Could you check a few things on this model? Use its own coordinates, in mm. A direction names the side the tool comes from. Round coordinates to 2 decimals unless told otherwise and drop trailing zeros. Write each loop counter-clockwise with the first axis right and the second up, starting at its lowest first coordinate (ties: lowest second). Pieces come first, ordered by that corner, then holes. Notation, with made-up numbers: M 6,18 L 47,18 A9 cw 47,26 Z; hole C 11,45.5 d5. An arc over 180 degrees is marked long. One line per item, written item: value. Start each with the question number.
(1) I want a section at B-B on y = 18. Please give me the cut outline in (x, z), and give its area (3 significant figures).
(2) If I drill on L1, parallel to Y at x = 4, z = 4.5; L2, parallel to Y at x = 10.5, z = 1.75, over which ranges is the centre line in solid material (lowest first)?
(3) I want a section at A-A on z = 5.25. Count the separate pieces of the cut face and the enclosed holes in it, and give its area (3 significant figures).
(4) I'm going to push a flat-ended pin straight in: pin 1 Ø1 at (x, y) = (-10, -40) entering from -Z. Where does the tip first touch, or does it pass through?
(5) Thinking about a two-plate mould opening in X: for faces 4 (the face through (-69.947, -1, 5)), 5 (the face through (-6, -74, 0)), 6 (the face through (72.986, -73.297, 6.19)), which applies, released by +X, released by -X, zero draft, split by the parting line, or undercut?
(6) Which directions (+Z, -Z, +X, -X, +Y, -Y) give clear straight access to the entire face, cutting with the end or side of a thin tool? Please do faces 1 (the face through (-78, -77, 6)), 2 (the face through (1, -69.947, 5)), 3 (the face through (77.552, -1, 6)).
```python
from build123d import *

# Parameters (mm, degrees)
F1_DEPTH = 10.5
F3_DEPTH = 10
F5_DEPTH = 9
F6_R     = 2


with BuildPart() as f1:
    # F0 (on Top) → F1 (new body)
    with BuildSketch(Plane.XY):
        with BuildLine():
            Line((-74, -79), (59, -79))
            ThreePointArc((59, -79), (73.1421356237, -73.1421356237), (79, -59))
            Line((79, -59), (79, 59))
            ThreePointArc((79, 59), (73.1421356237, 73.1421356237), (59, 79))
            Line((59, 79), (-59, 79))
            ThreePointArc((-59, 79), (-73.1421356237, 73.1421356237), (-79, 59))
            Line((-79, 59), (-79, -74))
            ThreePointArc((-79, -74), (-77.5355339059, -77.5355339059), (-74, -79))
        make_face()
    extrude(amount=F1_DEPTH)

    # F2 (on face) → F3 (cut)
    with BuildSketch(Plane.XY.offset(10.5)):
        with BuildLine():
            Line((77.5522068143, -59), (77.5522068143, 59))
            ThreePointArc((77.5522068143, 59), (72.1183912444, 72.1183912444), (59, 77.5522068143))
            Line((59, 77.5522068143), (-59, 77.5522068143))
            ThreePointArc((-59, 77.5522068143), (-72.1183912444, 72.1183912444), (-77.5522068143, 59))
            Line((-77.5522068143, 59), (-77.5522068143, -59.0002068143))
            ThreePointArc((-77.5522068143, -59.0002068143), (-72.1184518189, -72.1184518189), (-59.0002068143, -77.5522068143))
            Line((-59.0002068143, -77.5522068143), (59, -77.5522068143))
            ThreePointArc((59, -77.5522068143), (72.1183912444, -72.1183912444), (77.5522068143, -59))
        make_face()
        with BuildLine():
            ThreePointArc((59, 70.9469467402), (67.4477670544, 67.4477670544), (70.9469467402, 59))
            Line((70.9469467402, 59), (70.9469467402, -59))
            ThreePointArc((70.9469467402, -59), (67.4477670544, -67.4477670544), (59, -70.9469467402))
            Line((59, -70.9469467402), (-58.9999467402, -70.9469467402))
            ThreePointArc((-58.9999467402, -70.9469467402), (-67.447751455, -67.447751455), (-70.9469467402, -58.9999467402))
            Line((-70.9469467402, -58.9999467402), (-70.9469467402, 59))
            ThreePointArc((-70.9469467402, 59), (-67.4477670544, 67.4477670544), (-59, 70.9469467402))
            Line((-59, 70.9469467402), (59, 70.9469467402))
        make_face(mode=Mode.SUBTRACT)
    extrude(amount=-F3_DEPTH, mode=Mode.SUBTRACT)

    # F4 (on face) → F5 (cut)
    with BuildSketch(Plane(origin=(0, 0, 0), x_dir=(1, 0, 0), z_dir=(0, 0, -1))):
        with BuildLine():
            ThreePointArc((59, -69.9469467402), (66.7406602732, -66.7406602732), (69.9469467402, -59))
            Line((69.9469467402, -59), (69.9469467402, 59))
            ThreePointArc((69.9469467402, 59), (66.7406602732, 66.7406602732), (59, 69.9469467402))
            Line((59, 69.9469467402), (-58.9999467402, 69.9469467402))
            ThreePointArc((-58.9999467402, 69.9469467402), (-66.7406446738, 66.7406446738), (-69.9469467402, 58.9999467402))
            Line((-69.9469467402, 58.9999467402), (-69.9469467402, -59))
            ThreePointArc((-69.9469467402, -59), (-66.7406602732, -66.7406602732), (-59, -69.9469467402))
            Line((-59, -69.9469467402), (59, -69.9469467402))
        make_face()
    extrude(amount=-F5_DEPTH, mode=Mode.SUBTRACT)

    # F6
    f6_edges = [f1.edges().sort_by_distance(p)[0] for p in [
        (-7.5, -79, 0),
        (-77.535534, -77.535534, 0),
        (73.142136, -73.142136, 0),
        (-79, -7.5, 0),
        (79, 0, 0),
        (-73.142136, 73.142136, 0),
        (73.142136, 73.142136, 0),
        (0, 79, 0),
        (-69.946947, 2.7e-05, 0),
        (-66.740645, -66.740645, 0),
        (2.7e-05, -69.946947, 0),
        (66.74066, -66.74066, 0),
        (69.946947, 0, 0),
        (66.74066, 66.74066, 0),
        (0, 69.946947, 0),
        (-66.74066, 66.74066, 0),
        (-67.447767, 67.447767, 10.5),
        (0, 70.946947, 10.5),
        (67.447767, 67.447767, 10.5),
        (70.946947, 0, 10.5),
        (67.447767, -67.447767, 10.5),
        (2.7e-05, -70.946947, 10.5),
        (-67.447751, -67.447751, 10.5),
        (-70.946947, 2.7e-05, 10.5),
    ]]
    fillet(f6_edges, radius=F6_R)


solid = f1.part
```
Found:
1. outline: M -79,2 A2 ccw -77,0 L -71.95,0 A2 ccw -69.95,2 L -69.95,9 L 69.95,9 L 69.95,2 A2 ccw 71.95,0 L 77,0 A2 ccw 79,2 L 79,10.5 L 77.55,10.5 L 77.55,0.5 L 70.95,0.5 L 70.95,8.5 A2 ccw 68.95,10.5 L -68.95,10.5 A2 ccw -70.95,8.5 L -70.95,0.5 L -77.55,0.5 L -77.55,10.5 L -79,10.5 Z
1. area: 263 mm²
2. L1: y = -79 to -77.55, -70.95 to -69.95, 69.95 to 70.95, 77.55 to 79
2. L2: y = -78.98 to -77.55, -70.95 to -69.96, 69.96 to 70.95, 77.55 to 78.98
3. separate pieces: 2
3. enclosed holes: 2
3. area: 1,480 mm²
4. pin 1: stops at z = 9
5. face 4: undercut
5. face 5: zero draft
5. face 6: released by +X
6. face 1: +Z, -Z, -X, -Y
6. face 2: -Z
6. face 3: +Z
